from build123d import *

# Parameters (mm, degrees)
F0_W     = 50
F0_H     = 12
F1_DEPTH = 4
F2_R     = 4.1
F2_R_2   = 3.6
F3_DEPTH = 3
F4_DEPTH = 25
F5_R     = 5


with BuildPart() as f1:
    # F0 (on Top) → F1 (new body)
    with BuildSketch(Plane.XY):
        with Locations((5.119761, 6)):
            Rectangle(F0_W, F0_H)
    extrude(amount=F1_DEPTH)

    # F2 (on face) → F3 (cut)
    with BuildSketch(Plane.XY.offset(4)):
        with Locations((-14.880239, 6)):
            Circle(F2_R)
        with Locations((-14.880239, 6)):
            Circle(F2_R_2, mode=Mode.SUBTRACT)
        with Locations((5.119761, 6)):
            Circle(F2_R)
        with Locations((5.119761, 6)):
            Circle(F2_R_2, mode=Mode.SUBTRACT)
        with Locations((25.119761, 6)):
            Circle(F2_R)
        with Locations((25.119761, 6)):
            Circle(F2_R_2, mode=Mode.SUBTRACT)
    extrude(amount=-F3_DEPTH, mode=Mode.SUBTRACT)

    # F2 (on face) → F4 (cut)
    with BuildSketch(Plane.XY.offset(4)):
        with Locations((-14.880239, 6)):
            Circle(F2_R_2)
        with Locations((5.119761, 6)):
            Circle(F2_R_2)
        with Locations((25.119761, 6)):
            Circle(F2_R_2)
    extrude(amount=-F4_DEPTH, mode=Mode.SUBTRACT)

    # F5
    f5_edges = [f1.edges().sort_by_distance(p)[0] for p in [
        (30.119761, 12, 2),
        (30.119761, 0, 2),
        (-19.880239, 12, 2),
        (-19.880239, 0, 2),
    ]]
    fillet(f5_edges, radius=F5_R)


solid = f1.part
Can you work these out from the model? Positions are in its coordinate system, mm. A direction names the side the tool comes from. Coordinates: 2 decimals unless noted, no trailing zeros. Write each loop counter-clockwise with the first axis right and the second up, starting at its lowest first coordinate (ties: lowest second). Pieces come first, ordered by that corner, then holes. Notation, with made-up numbers: M -11.75,13 L 13.25,13 A16 cw 13.25,28 Z; hole C -9.75,86.25 d7. An arc over 180 degrees is marked long. Use one line per item in the form item = value.
Q1. If we section it at A-A (y = 6): Write out the boundary of the cut face in (x, z), then the cut area to 3 significant figures.
Model answer:
outline = M -19.88,0 L -18.48,0 L -18.48,1 L -18.98,1 L -18.98,4 L -19.88,4 Z; M -11.28,0 L 1.52,0 L 1.52,1 L 1.02,1 L 1.02,4 L -10.78,4 L -10.78,1 L -11.28,1 Z; M 8.72,0 L 21.52,0 L 21.52,1 L 21.02,1 L 21.02,4 L 9.22,4 L 9.22,1 L 8.72,1 Z; M 28.72,0 L 30.12,0 L 30.12,4 L 29.22,4 L 29.22,1 L 28.72,1 Z
area = 105 mm^2
Q2. If we section it at B-B (z = 2.85): Write out the boundary of the cut face in (x, y).
Model answer:
outline = M -19.88,5 A5 ccw -14.88,0 L 25.12,0 A5 ccw 30.12,5 L 30.12,7 A5 ccw 25.12,12 L -14.88,12 A5 ccw -19.88,7 Z; hole C -14.88,6 d8.2; hole C 5.12,6 d8.2; hole C 25.12,6 d8.2
Q3. If we section it at C-C (y = 8.25): Write out the boundary of the cut face in (x, z), then the cut area to 3 significant figures.
Model answer:
outline = M -19.72,0 L -17.69,0 L -17.69,1 L -18.31,1 L -18.31,4 L -19.72,4 Z; M -12.07,0 L 2.31,0 L 2.31,1 L 1.69,1 L 1.69,4 L -11.45,4 L -11.45,1 L -12.07,1 Z; M 7.93,0 L 22.31,0 L 22.31,1 L 21.69,1 L 21.69,4 L 8.55,4 L 8.55,1 L 7.93,1 Z; M 27.93,0 L 29.96,0 L 29.96,4 L 28.55,4 L 28.55,1 L 27.93,1 Z
area = 120 mm^2
Q4. For faces 1 (the cylindrical face through (-12.945, 9.036, 0.507)), 2 (the cylindrical face through (-11.093, 4.43, 2.521)), which set-ups out of +Z, -Z, +X, -X, +Y, -Y let a thin tool reach every point of the face, with its end or its side?
Model answer:
face_1 = +Z, -Z
face_2 = +Z
Q5. We'd pull the mould along X, two halves only. Please class faces 3 (the cylindrical face through (28.62, 1.43, 2.03)), 4 (the cylindrical face through (28.907, 4.43, 2.521)), 5 (the flat face through (-19.88, 6, 2)): +X half, -X half, draft (parallel to the pull), parting line (faces both ways), or undercut.
Model answer:
face_3 = +X half
face_4 = undercut
face_5 = -X half
Q6. If we section it at D-D (y = 11): Write out the boundary of the cut face in (x, z), then the cut area to 3 significant figures.
Model answer:
outline = M -17.88,0 L 28.12,0 L 28.12,4 L -17.88,4 Z
area = 184 mm^2
Q7. For P1, Ø2.5, axis at x = 7, y = 5, coming from the +Z side; P2, Ø1, axis at y = 9, z = 2.5, coming from the -X side, each with a flat end and sliding along its axis, tell me the tip position at first contact or that it passes through.
Model answer:
P1 = through
P2 = -19.65
Q8. I need wall thicknesses on line 1 along X through (y, z) = (7.75, 0.7); line 2 along X through (y, z) = (4, 0.5); line 3 along Z through (x, y) = (21.5, 7.5). Which ranges of each line are inside material? Lowest first, please. Write a range as from..to.
Model answer:
line_1 = -19.82..-18.03, -11.73..1.97, 8.27..21.97, 28.27..30.06
line_2 = -19.78..-17.87, -11.89..2.13, 8.11..22.13, 28.11..30.02
line_3 = 0..1
